Verification items for the finished model (mm, model axes). A direction names the side the tool comes from. Give positions to 0.01 mm unless a question says otherwise; leave off trailing zeros. Order: outer loops, then holes, each group sorted by start corner. A loop starts at its lowest first (then second) coordinate and runs counter-clockwise, first axis right, second up. Notation, with made-up numbers: M -33.5,37.25 L -2.5,37.25 A20 ccw -2.5,72.25 Z; hole C 13,-20 d5. An arc over 180 degrees is marked long. Answer as a JSON object with one key per item and string values.
Autodesk Inventor part; units mm, degrees
ref_plane "YZ Plane" through (0, 0, 0) normal (1, 0, 0) x (0, 1, 0)
ref_plane "XZ Plane" through (0, 0, 0) normal (0, 1, 0) x (-1, 0, 0)
ref_plane "XY Plane" through (0, 0, 0) normal (0, 0, 1) x (1, 0, 0)
sketch "Náčrt1" plane through (0, 0, 0) normal (0, 0, 1) x (1, 0, 0)
  line L0 (0, 0) -> (100, 0)
  line L1 (100, 0) -> (100, 50)
  line L2 (100, 50) -> (0, 50)
  line L3 (0, 50) -> (0, 0)
  dimension "d0" = 100
  dimension "d1" = 50
extrude "Vysunutí1" add sketch "Náčrt1" along normal blind 49
sketch "Náčrt2" plane through (0, 0, 49) normal (0, 0, 1) x (1, 0, 0)
  line L0 (2, 2) -> (98, 2)
  line L1 (98, 2) -> (98, 48)
  line L2 (98, 48) -> (2, 48)
  line L3 (2, 48) -> (2, 2)
  point P0 (0, 0)
  dimension "d4" = 96
  dimension "d5" = 46
extrude "Vysunutí2" cut sketch "Náčrt2" against normal blind 48
sketch "Náčrt3" plane through (0, 0, 1) normal (0, 0, 1) x (1, 0, 0)
  circle A0 centre (10, 10) radius 4
  line L0 (98, 48) -> (98, 2)
  line L1 (2, 48) -> (98, 48)
  line L2 (2, 2) -> (2, 48)
  line L3 (98, 2) -> (2, 2)
  circle A1 centre (10, 40) radius 4
  circle A2 centre (90, 10) radius 4
  circle A3 centre (90, 40) radius 4
  line L4 (98, 2) -> (2, 2)
  line L5 (50, 25) -> (2, 2)
  point P0 (0, 0)
  point P1 (10.387, 6.0188)
  point P2 (12.8605, 7.204)
  dimension "d8" = 8
  dimension "d11" = 30
  dimension "d14" = 80
  dimension "d19" = 25.602
  dimension "d20" = 40
  dimension "d22" = 15
  dimension "d23" = 48
extrude "Vysunutí3" add sketch "Náčrt3" along normal blind 36.5 contours A0 L5 | A1 | A2 | A3 picked at (11.6868, 9.0428)
hole "Díra1" at (10.0461, 9.9039, 37.5) direction (0, 0, -1) diameter 2.459 end through all
sketch "Náčrt4" plane through (0, 0, 0) normal (0, 0, -1) x (-1, 0, 0)
  point P0 (0, 0)
hole "Díra2" at (90, 40, 37.5) direction (0, 0, -1) diameter 2.459 end through all
hole "Díra3" at (90, 10, 37.5) direction (0, 0, -1) diameter 2.459 end through all
hole "Díra4" at (10, 40, 37.5) direction (0, 0, -1) diameter 2.459 end through all
equation "\"d22\" = 0.5 * d11"
properties part number "bottom"
Q1. Section check D-D on x = 32. Record the cut outline in (y, z).
Resolved:
{"outline": "M 0,0 L 50,0 L 50,49 L 48,49 L 48,1 L 2,1 L 2,49 L 0,49 Z"}
Q2. Section check A-A on y = 40. Record the cut outline in (x, z), then the cut area to 3 significant figures.
Resolved:
{"outline": "M 0,0 L 8.77,0 L 8.77,37.5 L 6,37.5 L 6,1 L 2,1 L 2,49 L 0,49 Z; M 11.23,0 L 88.77,0 L 88.77,37.5 L 86,37.5 L 86,1 L 14,1 L 14,37.5 L 11.23,37.5 Z; M 91.23,0 L 100,0 L 100,49 L 98,49 L 98,1 L 94,1 L 94,37.5 L 91.23,37.5 Z", "area": "692 mm²"}
Q3. Tool access check on faces 1 (the face through (9.479, 36.034, 18.994)), 2 (the face through (49, 0, 24)). Record the directions out of +Z, -Z, +X, -X, +Y, -Y that give a thin tool (end or side, any length) a straight path to the whole face; none if there is none.
Resolved:
{"face 1": "+Z", "face 2": "+Z, -Z, +X, -X, -Y"}
Q4. Material ranges on L1, parallel to X at y = 36.5, z = 25; L2, parallel to X at y = 29.5, z = 27.5; L3, parallel to Y at x = 24, z = 40.5, recorded low to high.
Resolved:
{"L1": "x = 0 to 2, 8.06 to 11.94, 88.06 to 91.94, 98 to 100", "L2": "x = 0 to 2, 98 to 100", "L3": "y = 0 to 2, 48 to 50"}
Q5. Release check for a two-part mould opening along X. For faces 3 (the face through (0, 25, 24)), 4 (the face through (49, 25, 1)), 5 (the face through (35, 1, 49)) record: +X half, -X half, draft (parallel to the pull), parting line (faces both ways), or undercut.
Resolved:
{"face 3": "-X half", "face 4": "undercut", "face 5": "draft"}
Q6. Gauge pin test, flat ends, axial feed: pin 1 Ø4 at (x, y) = (11.5, 8.5) entering from +Z; pin 2 Ø2 at (x, y) = (10, 40) entering from +Z; pin 3 Ø2 at (x, y) = (42, 7.5) entering from +Z. Record the tip position at first contact, or that the pin passes through.
Resolved:
{"pin 1": "stops at z = 37.5", "pin 2": "passes through", "pin 3": "stops at z = 1"}
Q7. Section check C-C on z = 29. Count the separate pieces of the cut face and the enclosed holes in it, then the cut area to 3 significant figures.
Resolved:
{"separate pieces": "5", "enclosed holes": "5", "area": "766 mm²"}
Q8. Section check B-B on x = 90. Record the cut outline in (y, z), then the cut area to 3 significant figures.
Resolved:
{"outline": "M 0,0 L 8.77,0 L 8.77,37.5 L 6,37.5 L 6,1 L 2,1 L 2,49 L 0,49 Z; M 11.23,0 L 38.77,0 L 38.77,37.5 L 36,37.5 L 36,1 L 14,1 L 14,37.5 L 11.23,37.5 Z; M 41.23,0 L 50,0 L 50,49 L 48,49 L 48,1 L 44,1 L 44,37.5 L 41.23,37.5 Z", "area": "642 mm²"}
